Could you check a few things on this model? Use its own coordinates, in mm. Coordinates: 2 decimals unless noted, no trailing zeros. Order: outer loops, then holes, each group sorted by start corner. A loop starts at its lowest first (then second) coordinate and runs counter-clockwise, first axis right, second up.
```python
from build123d import *

# Parameters (mm, degrees)
SKETCH2_W                       = 185.42
SKETCH2_H                       = 223.52
SKETCH2_R                       = 2.5527
BOSS_EXTRUDE1_DEPTH             = 6.35
FILLET2_R                       = 6.35
SKETCH5_R                       = 4.445
CUT_EXTRUDE3_DEPTH              = 146.347047442
SKETCH6_R                       = 3.2639
CUT_EXTRUDE6_DEPTH              = 146.347047442
SKETCH8_R                       = 6.35
CUT_EXTRUDE7_DEPTH              = 146.347047442
F_55_0_052_DIAMETER_HOLE1_D     = 1.3208
F_55_0_052_DIAMETER_HOLE2_D     = 1.3208
F_55_0_052_DIAMETER_HOLE2_DEPTH = 25.4
F_55_0_052_DIAMETER_HOLE2_TIP   = 0.396808353


with BuildPart() as part:
    # Sketch2 → Boss-Extrude1 (new body)
    with BuildSketch(Plane.XY.offset(6.35)):
        Rectangle(SKETCH2_W, SKETCH2_H)
        with Locations((-19.05, 101.6)):
            Circle(SKETCH2_R, mode=Mode.SUBTRACT)
        with Locations((19.05, 101.6)):
            Circle(SKETCH2_R, mode=Mode.SUBTRACT)
        with Locations((-19.05, -101.6)):
            Circle(SKETCH2_R, mode=Mode.SUBTRACT)
        with Locations((19.05, -101.6)):
            Circle(SKETCH2_R, mode=Mode.SUBTRACT)
    extrude(amount=BOSS_EXTRUDE1_DEPTH)

    # Fillet2
    fillet2_edges = [part.edges().sort_by_distance(p)[0] for p in [
        (-92.71, 111.76, 9.525),
        (92.71, 111.76, 9.525),
        (92.71, -111.76, 9.525),
        (-92.71, -111.76, 9.525),
    ]]
    fillet(fillet2_edges, radius=FILLET2_R)

    # Sketch5 → Cut-Extrude3 (cut, through all)
    with BuildSketch(Plane.XY.offset(12.7)):
        with Locations((0, 92.71)):
            Circle(SKETCH5_R)
    extrude(amount=-CUT_EXTRUDE3_DEPTH, mode=Mode.SUBTRACT)

    # Sketch6 → Cut-Extrude6 (cut, through all)
    with BuildSketch(Plane(origin=(0, 0, 6.35), x_dir=(-1, 0, 0), z_dir=(0, 0, -1))):
        with Locations((-79.375, -80.01)):
            Circle(SKETCH6_R)
        with Locations(Location((79.375, -80.01, 0), (0, 0, 180))):
            Circle(SKETCH6_R)
        with Locations((-79.375, -99.06)):
            Circle(SKETCH6_R)
        with Locations(Location((79.375, -99.06, 0), (0, 0, 180))):
            Circle(SKETCH6_R)
    extrude(amount=-CUT_EXTRUDE6_DEPTH, mode=Mode.SUBTRACT)

    # Sketch8 → Cut-Extrude7 (cut, through all)
    with BuildSketch(Plane.XY.offset(12.7)):
        with Locations((0, 35.306)):
            Circle(SKETCH8_R)
        with Locations((57.15, -82.55)):
            Circle(SKETCH8_R)
        with Locations((19.05, -82.55)):
            Circle(SKETCH8_R)
        with Locations((-19.05, -82.55)):
            Circle(SKETCH8_R)
        with Locations((-57.15, -82.55)):
            Circle(SKETCH8_R)
        with BuildLine():
            Line((63.5, -36.068), (57.15, -36.068))
            ThreePointArc((57.15, -36.068), (55.5625, -34.4805), (57.15, -32.893))
            Line((57.15, -32.893), (63.5, -32.893))
            ThreePointArc((63.5, -32.893), (65.0875, -34.4805), (63.5, -36.068))
        make_face()
        with BuildLine():
            Line((-57.15, -36.068), (-63.5, -36.068))
            ThreePointArc((-63.5, -36.068), (-65.0875, -34.4805), (-63.5, -32.893))
            Line((-63.5, -32.893), (-57.15, -32.893))
            ThreePointArc((-57.15, -32.893), (-55.5625, -34.4805), (-57.15, -36.068))
        make_face()
        with BuildLine():
            Line((-57.15, -73.66), (-63.5, -73.66))
            ThreePointArc((-63.5, -73.66), (-65.0875, -72.0725), (-63.5, -70.485))
            Line((-63.5, -70.485), (-57.15, -70.485))
            ThreePointArc((-57.15, -70.485), (-55.5625, -72.0725), (-57.15, -73.66))
        make_face()
        with BuildLine():
            Line((57.15, -70.485), (63.5, -70.485))
            ThreePointArc((63.5, -70.485), (65.0875, -72.0725), (63.5, -73.66))
            Line((63.5, -73.66), (57.15, -73.66))
            ThreePointArc((57.15, -73.66), (55.5625, -72.0725), (57.15, -70.485))
        make_face()
    extrude(amount=-CUT_EXTRUDE7_DEPTH, mode=Mode.SUBTRACT)

    # #55 (0.052) Diameter Hole1 (through all)
    with Locations(Plane.XY.offset(12.7)):
        with Locations((-13.5636, 35.069031778), (-44.0436, 35.069031778), (-57.3786, 35.069031778), (-44.0436, 69.409831778), (-87.8586, 35.069031778), (-87.8586, 69.409831778)):
            Hole(F_55_0_052_DIAMETER_HOLE1_D / 2)

    # #55 (0.052) Diameter Hole2
    with Locations(Plane.XY.offset(12.7)):
        with Locations((6.08, 48.508231778), (6.08, 76.508231778), (58.43, 82.208231778), (56.93, 33.508231778)):
            Hole(F_55_0_052_DIAMETER_HOLE2_D / 2, depth=F_55_0_052_DIAMETER_HOLE2_DEPTH)
            with Locations((0, 0, -(F_55_0_052_DIAMETER_HOLE2_DEPTH + F_55_0_052_DIAMETER_HOLE2_TIP / 2))):  # 118° drill point
                Cone(0, F_55_0_052_DIAMETER_HOLE2_D / 2, F_55_0_052_DIAMETER_HOLE2_TIP, mode=Mode.SUBTRACT)


solid = part.part
```
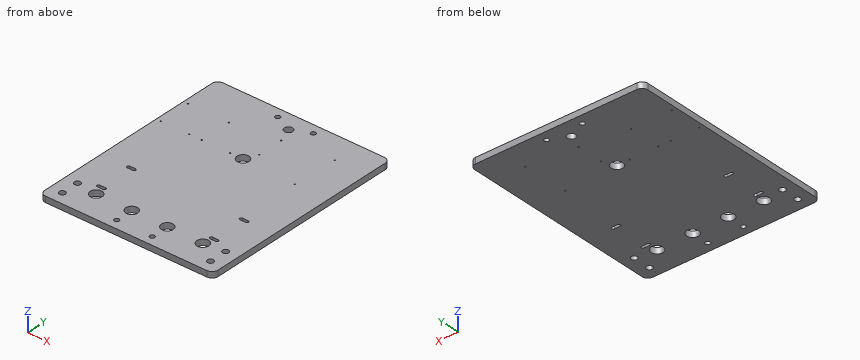
Item 1: Suppose I cut it at A-A (x = -61). List the corners of the cut face in (y, z) for me (3 decimals).
Item 2: I need wall thicknesses on line 1 (Y direction, x = 0, z = 9) (3 decimals); line 2 (Y direction, x = 56.93, z = 10.5); line 3 (Y direction, x = -19.05, z = 8.25). Which ranges of each line are inside material? Lowest first, please.
Item 3: Suppose I cut it at C-C (z = 9). Count the separate pieces of the cut face and the enclosed holes in it, and give its area (3 significant figures).
Item 4: Suppose I cut it at B-B (y = -80.01). List the corners of the cut face in (x, z) for me.
Geometry results:
1. outline: (-111.76, 6.35) - (-87.6, 6.35) - (-87.6, 12.7) - (-111.76, 12.7) - close; (-77.5, 6.35) - (-73.66, 6.35) - (-73.66, 12.7) - (-77.5, 12.7) - close; (-70.485, 6.35) - (-36.068, 6.35) - (-36.068, 12.7) - (-70.485, 12.7) - close; (-32.893, 6.35) - (111.76, 6.35) - (111.76, 12.7) - (-32.893, 12.7) - close
2. line 1: y = -111.76 to 28.956, 41.656 to 88.265, 97.155 to 111.76
2. line 2: y = -111.76 to -88.9, -76.2 to -73.64, -70.5 to -36.05, -32.91 to 32.85, 34.17 to 111.76
2. line 3: y = -111.76 to -104.15, -99.05 to -88.9, -76.2 to 99.05, 104.15 to 111.76
3. separate pieces: 1
3. enclosed holes: 28
3. area: 40,400 mm2
4. outline: (-92.71, 6.35) - (-82.64, 6.35) - (-82.64, 12.7) - (-92.71, 12.7) - close; (-76.11, 6.35) - (-62.97, 6.35) - (-62.97, 12.7) - (-76.11, 12.7) - close; (-51.33, 6.35) - (-24.87, 6.35) - (-24.87, 12.7) - (-51.33, 12.7) - close; (-13.23, 6.35) - (13.23, 6.35) - (13.23, 12.7) - (-13.23, 12.7) - close; (24.87, 6.35) - (51.33, 6.35) - (51.33, 12.7) - (24.87, 12.7) - close; (62.97, 6.35) - (76.11, 6.35) - (76.11, 12.7) - (62.97, 12.7) - close; (82.64, 6.35) - (92.71, 6.35) - (92.71, 12.7) - (82.64, 12.7) - close
